```python
from build123d import *

# Parameters (mm, degrees)
F0_R      = 7.35
F1_DEPTH  = 5.842
F2_R      = 2
F3_W      = 3.0988
F3_H      = 6.35
F4_DEPTH  = 25.4
F5_W      = 12.7
F5_H      = 3.0988
F6_DEPTH  = 5.842
F8_DEPTH  = 5.842
F10_DEPTH = 25.4
F11_R     = 1.5


with BuildPart() as f1:
    # F0 (on Front) → F1 (new body)
    with BuildSketch(Plane.XZ):
        Polygon((31.75, 11.1125), (-31.75, 11.1125), (-31.75, -11.1125), (-11.43, -11.1125), (-7.62, -1.5875), (0, -1.5875), (7.62, -1.5875), (11.43, -11.1125), (31.75, -11.1125), align=None)
        with Locations((-19.05, 0)):
            Circle(F0_R, mode=Mode.SUBTRACT)
        with Locations((19.05, 0)):
            Circle(F0_R, mode=Mode.SUBTRACT)
    extrude(amount=F1_DEPTH)

    # F2
    f2_edges = [f1.edges().sort_by_distance(p)[0] for p in [
        (-11.43, -2.921, -11.1125),
        (-7.62, -2.921, -1.5875),
        (7.62, -2.921, -1.5875),
        (11.43, -2.921, -11.1125),
    ]]
    fillet(f2_edges, radius=F2_R)

    # F3 (on face) → F4 (cut)
    with BuildSketch(Plane(origin=(0, 0, 0), x_dir=(-1, 0, 0), z_dir=(0, 1, 0))):
        with Locations((4.7625, 4.7625)):
            Rectangle(F3_W, F3_H)
    extrude(amount=-F4_DEPTH, mode=Mode.SUBTRACT)

    # F5 (on face) → F6 (join, through all)
    with BuildSketch(Plane.XZ.offset(5.842)):
        with Locations((-12.7, 12.6619)):
            Rectangle(F5_W, F5_H)
        with Locations((12.7, 12.6619)):
            Rectangle(F5_W, F5_H)
    extrude(amount=-F6_DEPTH)

    # F7 (on face) → F8 (join, through all)
    with BuildSketch(Plane.XZ.offset(5.842)):
        Polygon((38.592, 6.35), (32.75, 6.35), (32.75, 11.1125), (31.75, 11.1125), (31.75, 6.35), (31.75, -6.35), (31.75, -11.1125), (32.75, -11.1125), (32.75, -6.35), (38.592, -6.35), align=None)
        Polygon((-31.75, 6.35), (-31.75, 11.1125), (-32.75, 11.1125), (-32.75, 6.35), (-38.592, 6.35), (-38.592, -6.35), (-32.75, -6.35), (-32.75, -11.1125), (-31.75, -11.1125), (-31.75, -6.35), align=None)
    extrude(amount=-F8_DEPTH)

    # F9 (on face) → F10 (cut)
    with BuildSketch(Plane.XZ.offset(5.842)):
        with BuildLine():
            Line((-22.22424, -11.1125), (-22.22424, -8.5725))
            ThreePointArc((-22.22424, -8.5725), (-24.0500663267, -7.652639581), (-25.625793171, -6.35))
            Line((-25.625793171, -6.35), (-32.75, -6.35))
            Line((-32.75, -6.35), (-32.75, -8.5725))
            Line((-32.75, -8.5725), (-32.75, -11.1125))
            Line((-32.75, -11.1125), (-22.22424, -11.1125))
        make_face()
        with BuildLine():
            Line((32.75, -8.5725), (32.75, -6.35))
            Line((32.75, -6.35), (25.625793171, -6.35))
            ThreePointArc((25.625793171, -6.35), (24.0500663267, -7.652639581), (22.22424, -8.5725))
            Line((22.22424, -8.5725), (22.22424, -11.1125))
            Line((22.22424, -11.1125), (32.75, -11.1125))
            Line((32.75, -11.1125), (32.75, -8.5725))
        make_face()
    extrude(amount=-F10_DEPTH, mode=Mode.SUBTRACT)

    # F11
    f11_edges = [f1.edges().sort_by_distance(p)[0] for p in [
        (25.625793, -2.921, -6.35),
        (22.22424, -2.921, -11.1125),
        (22.22424, -2.921, -8.5725),
        (-25.625793, -2.921, -6.35),
        (-22.22424, -2.921, -8.5725),
        (-22.22424, -2.921, -11.1125),
    ]]
    fillet(f11_edges, radius=F11_R)


solid = f1.part
```
Model file for the job. Use its own axes, mm. A direction names the side the tool comes from. Coordinates: 2 decimals unless noted, no trailing zeros. Loops run counter-clockwise (first coordinate to the right, second up) from the corner with the lowest first, then second, coordinate; pieces in that order, holes last. Notation, with made-up numbers: (-8, -21) - (39, -21) arc R13 cw to (39, 0) - close; hole circle Ø7 at (53, 20). An arc over 180 degrees is marked (long way). Write item = value, one per line. Start each with the question number.
Item 1: Drop flat-ended pins along their axis: pin 1 Ø1.4 at (y, z) = (-2, 9) entering from -X; pin 2 Ø0.9 at (y, z) = (-3, 13) entering from +X; pin 3 Ø1 at (x, y) = (22.5, -3.5) entering from -Z. Give the stop position or say it passes through.
Item 2: Saw through at C-C, the plane y = -5.05. State how many separate pieces and enclosed holes the cut face has, then the cut area to 3 significant figures.
Item 3: Saw through at D-D, the plane z = 9.5. List the corners of the cut face in (x, y).
Item 4: Pull direction X, two halves, no side cores. Call faces 5 (the face through (7.4, -2.96, -1.94)), 6 (the face through (32.75, -3, 9)), 7 (the face through (36, -3, 6.35)): +X half, -X half, draft (parallel to the pull), parting line (faces both ways), or undercut.
Item 5: Saw through at A-A, the plane z = 0. List the corners of the cut face in (x, y), then the cut area to 3 significant figures.
Item 6: Wall check: probe 1 along X at (y, z) = (-5, 7.5); probe 2 along X at (y, z) = (-0.85, 6.5); probe 3 along Z at (x, y) = (-4.5, -2.15). Give the ranges that are in metal, low to high. Write a range as [from, to].
Item 7: 3-axis set-ups, long thin cutter, end or side, ignore diameter. For faces 1 (the face through (32, -3, -6.35)), 2 (the face through (19.05, -3, 13)), 3 (the face through (-19.05, -3, 13)), 4 (the face through (9.505, -2.88, -6.301)): which of +Z, -Z, +X, -X, +Y, -Y reach the whole face in a straight line?
Item 8: Saw through at B-B, the plane x = 17. List the corners of the cut face in (y, z), then the cut area to 3 significant figures.
Answers:
q1.pin_1 = -32.75
q1.pin_2 = 19.05
q1.pin_3 = -10.4
q2.separate_pieces = 1
q2.enclosed_holes = 3
q2.area = 1,050 mm2
q3.outline = (-32.75, -5.84) - (32.75, -5.84) - (32.75, 0) - (-32.75, 0) - close
q4.face_5 = undercut
q4.face_6 = +X half
q4.face_7 = draft
q5.outline = (-38.59, -5.84) - (-26.4, -5.84) - (-26.4, 0) - (-38.59, 0) - close; (-11.7, -5.84) - (11.7, -5.84) - (11.7, 0) - (-11.7, 0) - close; (26.4, -5.84) - (38.59, -5.84) - (38.59, 0) - (26.4, 0) - close
q5.area = 279 mm2
q6.probe_1 = [-32.75, -6.31], [-3.21, 32.75]
q6.probe_2 = [-32.75, -22.48], [-15.62, -6.31], [-3.21, 15.62], [22.48, 32.75]
q6.probe_3 = [-1.59, 1.59], [7.94, 11.11]
q7.face_1 = -Z, +X, +Y, -Y
q7.face_2 = +Z, +X, +Y, -Y
q7.face_3 = +Z, -X, +Y, -Y
q7.face_4 = -Z, +Y, -Y
q8.outline = (-5.84, -11.11) - (0, -11.11) - (0, -7.06) - (-5.84, -7.06) - close; (-5.84, 7.06) - (0, 7.06) - (0, 14.21) - (-5.84, 14.21) - close
q8.area = 65.5 mm2
